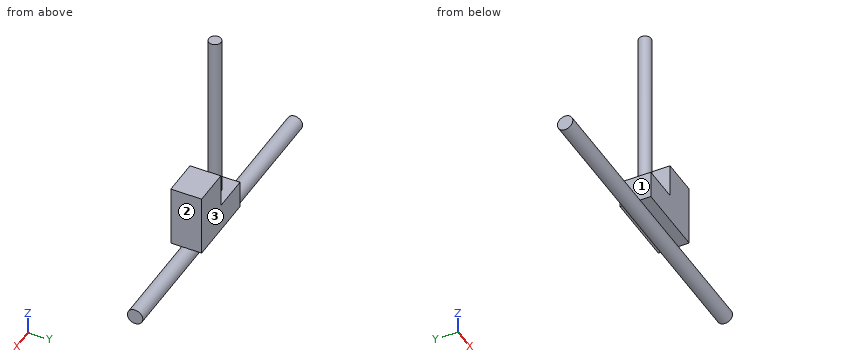
Solid Edge part; units mm, degrees
sketch "Sketch1" plane through (0, 0, 0) normal (0, 0, 1) x (1, 0, 0)
  line L0 (-12, -5) -> (12, -5)
  line L1 (12, -5) -> (12, 5)
  line L2 (12, 5) -> (-12, 5)
  line L3 (-12, 5) -> (-12, -5)
extrude "Protrusion1" add sketch "Sketch1" along normal blind 9
sketch "Sketch2" plane through (0, 0, 9) normal (0, 0, 1) x (1, 0, 0)
  line L0 (12, 5) -> (12, -5)
  line L1 (12, -5) -> (0, -5)
  line L2 (0, -5) -> (0, 5)
  line L3 (0, 5) -> (12, 5)
extrude "Wyciągnięcie_2" add sketch "Sketch2" along normal blind 11
sketch "Sketch3" plane through (-6, 0, 9) normal (0, 0, 1) x (1, 0, 0)
  circle A0 centre (0, 0) radius 2
extrude "Wyciągnięcie_3" add sketch "Sketch3" along normal blind 55
cosmetic_thread "Thread1"
sketch "Sketch4" plane through (-6, 0, 4.5) normal (-1, 0, 0) x (0, 1, 0)
  circle A0 centre (0, 6.95) radius 2.5
extrude "Wyciągnięcie_6" add sketch "Sketch4" along normal mid plane 100
Can you work these out from the model? Positions are in its coordinate system, mm. Face numbers are marked on the shaded views. A direction names the side the tool comes from. Coordinates: 2 decimals unless noted, no trailing zeros. Write each loop counter-clockwise with the first axis right and the second up, starting at its lowest first coordinate (ties: lowest second). Pieces come first, ordered by that corner, then holes. Notation, with made-up numbers: (-9.5, 76) -> (47.5, 76) arc R20 cw to (47.5, 107) -> close; hole circle Ø10 at (27.25, -39.75). An arc over 180 degrees is marked (long way). Write item = value, one per line.
(1) Imagine slicing it at D-D (x = 7.5). Please give me the cut outline in (y, z).
Verdict:
outline = (-5, 0) -> (-0.5, 0) arc R2.5 ccw (long way) to (0.5, 0) -> (5, 0) -> (5, 20) -> (-5, 20) -> close
(2) If I drill on probe 1 along Z at (x, y) = (4, -1); probe 2 along X at (y, z) = (-1.5, 13); probe 3 along Z at (x, y) = (-10, 1), over which ranges is the centre line in solid material (lowest first)?
Verdict:
probe_1 = -4.74 to -0.16, 0 to 20
probe_2 = -7.32 to -4.68, 0 to 12
probe_3 = -4.74 to -0.16, 0 to 9
(3) For pin 1 (1 mm diameter, centred on y = -3.5, z = 12, fed in from -X); pin 2 (1.5 mm diameter, centred on x = 3.5, y = 2, fed in from -Z); pin 3 (1.4 mm diameter, centred on x = 0.5, y = -3.5, fed in from -Z), each with a flat end and sliding along its axis, tell me the tip position at first contact or that it passes through.
Verdict:
pin_1 = 0
pin_2 = -4.62
pin_3 = 0
(4) Imagine slicing it at C-C (y = -3.75). Please give me the cut outline in (x, z).
Verdict:
outline = (-12, 0) -> (12, 0) -> (12, 20) -> (0, 20) -> (0, 9) -> (-12, 9) -> close
(5) Imagine slicing it at A-A (x = -6). Please give me the cut outline in (y, z).
Verdict:
outline = (-5, 0) -> (-0.5, 0) arc R2.5 ccw (long way) to (0.5, 0) -> (5, 0) -> (5, 9) -> (2, 9) -> (2, 64) -> (-2, 64) -> (-2, 9) -> (-5, 9) -> close
(6) On a 3-axis mill with a long thin cutter (end or side, diameter ignored), from which of +Z, -Z, +X, -X, +Y, -Y can I reach the whole of each face in a straight line? I mean the marked faces 1, 2 and 3. Say none if no direction works.
Verdict:
face_1 = +Z, -X, +Y, -Y
face_2 = +Z, +X, +Y, -Y
face_3 = +Z, -Z, +X, -X, +Y
(7) Imagine slicing it at B-B (z = -2.45). Please give me the cut outline in (x, y).
Verdict:
outline = (-56, -2.5) -> (44, -2.5) -> (44, 2.5) -> (-56, 2.5) -> close
